Read the model definition and answer for the solid it produces. Units are mm, in the model's axes. Face numbers are marked on the shaded views. A direction names the side the tool comes from. Coordinates: 2 decimals unless noted, no trailing zeros. Loops run counter-clockwise (first coordinate to the right, second up) from the corner with the lowest first, then second, coordinate; pieces in that order, holes last. Notation, with made-up numbers: (10, -6.5) -> (60, -6.5) arc R13 ccw to (60, 3.5) -> close; hole circle Ø1 at (-31, -17.75). An arc over 180 degrees is marked (long way). Answer as CSV lines item,"result".
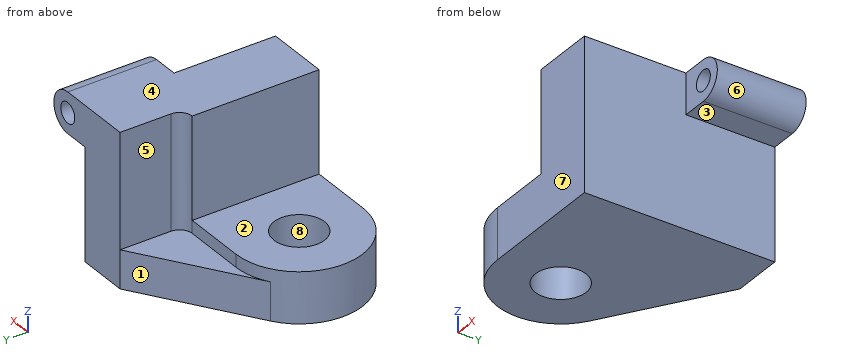
```python
from build123d import *

# Parameters (mm, degrees)
SKETCH1_R           = 10
BOSS_EXTRUDE1_DEPTH = 20
BOSS_EXTRUDE2_START = 20
BOSS_EXTRUDE2_DEPTH = 40
BOSS_EXTRUDE3_DEPTH = 15
SKETCH2_R           = 4
BOSS_EXTRUDE4_DEPTH = 35


with BuildPart() as part:
    # Sketch1 → Boss-Extrude1 (new body)
    with BuildSketch(Plane.XY):
        with BuildLine():
            ThreePointArc((0, -25), (-25, 0), (0, 25))
            Line((0, 25), (25, 25))
            Line((25, 25), (25, -25))
            Line((25, -25), (0, -25))
        make_face()
        Circle(SKETCH1_R, mode=Mode.SUBTRACT)
        with BuildLine():
            ThreePointArc((30, 30), (28.535533906, 26.464466094), (25, 25))
            Line((25, 25), (25, -25))
            Line((25, -25), (50, -25))
            Line((50, -25), (50, 15))
            Line((50, 15), (50, 50))
            Line((50, 50), (30, 50))
            Line((30, 50), (30, 30))
        make_face()
    extrude(amount=BOSS_EXTRUDE1_DEPTH)

    # Sketch1<3> → Boss-Extrude2 (add)
    with BuildSketch(Plane.XY.offset(BOSS_EXTRUDE2_START)):
        with BuildLine():
            ThreePointArc((30, 30), (28.535533906, 26.464466094), (25, 25))
            Line((25, 25), (25, -25))
            Line((25, -25), (50, -25))
            Line((50, -25), (50, 15))
            Line((50, 15), (50, 50))
            Line((50, 50), (30, 50))
            Line((30, 50), (30, 30))
        make_face()
    extrude(amount=BOSS_EXTRUDE2_DEPTH)

    # Sketch1<4> → Boss-Extrude3 (add)
    with BuildSketch(Plane.XY):
        with BuildLine():
            ThreePointArc((-13.852304693, 20.811382816), (-7.2358631, 23.929945365), (0, 25))
            Line((0, 25), (25, 25))
            ThreePointArc((25, 25), (28.535533906, 26.464466094), (30, 30))
            Line((30, 30), (30, 50))
            Line((30, 50), (-13.852304693, 20.811382816))
        make_face()
    extrude(amount=BOSS_EXTRUDE3_DEPTH)

    # Sketch2 → Boss-Extrude4 (add)
    with BuildSketch(Plane(origin=(0, 50, 0), x_dir=(1, 0, 0), z_dir=(0, 1, 0))):
        with BuildLine():
            Line((60, -44), (50, -44))
            Line((50, -44), (50, -60))
            Line((50, -60), (60, -60))
            ThreePointArc((60, -60), (68, -52), (60, -44))
        make_face()
        with Locations((60, -52)):
            Circle(SKETCH2_R, mode=Mode.SUBTRACT)
    extrude(amount=-BOSS_EXTRUDE4_DEPTH)


solid = part.part
```
Q1. Given pin 1 Ø10 at (y, z) = (12.5, 30.5) entering from +X; pin 2 Ø18 at (y, z) = (28, 41) entering from +X; pin 3 Ø2 at (y, z) = (21, 52.5) entering from -X; pin 4 Ø8 at (x, y) = (53, 29) entering from -Z, each flat-ended and moving along its own axis, determine where each tip first touches the part or whether it passes through.
Results:
pin 1,"stops at x = 50"
pin 2,"stops at x = 67.75"
pin 3,"stops at x = 25"
pin 4,"stops at z = 0"
Q2. A cutting plane is placed at B-B, the plane y = 0. Write down the section's boundary in (x, z).
Results:
outline,"(-25, 0) -> (-10, 0) -> (-10, 20) -> (-25, 20) -> close; (10, 0) -> (50, 0) -> (50, 60) -> (25, 60) -> (25, 20) -> (10, 20) -> close"
Q3. A cutting plane is placed at C-C, the plane z = 30.5. Write down the section's boundary in (x, y).
Results:
outline,"(25, -25) -> (50, -25) -> (50, 50) -> (30, 50) -> (30, 30) arc R5 cw to (25, 25) -> close"
Q4. A cutting plane is placed at A-A, the plane z = 52. Write down the section's boundary in (x, y).
Results:
outline,"(25, -25) -> (50, -25) -> (50, 15) -> (56, 15) -> (56, 50) -> (30, 50) -> (30, 30) arc R5 cw to (25, 25) -> close; (64, 15) -> (68, 15) -> (68, 50) -> (64, 50) -> close"
Q5. For the marked faces 1, 2, 3, 4 and 5, determine the directions among +Z, -Z, +X, -X, +Y, -Y from which every point of the face is accessible in a straight line to the end or side of a thin tool.
Results:
face 1,"+Z, -Z, -X, +Y"
face 2,"+Z, -X, +Y, -Y"
face 3,"-Z, +X, +Y, -Y"
face 4,"+Z, +X, -X, +Y, -Y"
face 5,"+Z, -X, +Y"
Q6. A cutting plane is placed at D-D, the plane y = -20. Write down the section's boundary in (x, z), and give its area (3 significant figures).
Results:
outline,"(-15, 0) -> (50, 0) -> (50, 60) -> (25, 60) -> (25, 20) -> (-15, 20) -> close"
area,"2,300 mm²"
Q7. Find the intervals of material crossed by probe 1 along Y at (x, z) = (0, 15.5); probe 2 along X at (y, z) = (40, 52); probe 3 along Z at (x, y) = (60, 42.5), in increasing order. Write a range as [from, to].
Results:
probe 1,"y = [-25, -10], [10, 25]"
probe 2,"x = [30, 56], [64, 68]"
probe 3,"z = [44, 48], [56, 60]"
Q8. For a pull along X with two mould halves and no side action, classify the marked faces 6, 7 and 8 as pulls with the +X half, pulls with the -X half, needs draft (parallel to the pull), parting line crosses it, or undercut.
Results:
face 6,"pulls with the +X half"
face 7,"needs draft"
face 8,"undercut"
